Geometry: final body of the model. Coordinates: model frame, mm. Give positions to 0.01 mm unless a question says otherwise; leave off trailing zeros. Write each loop counter-clockwise with the first axis right and the second up, starting at its lowest first coordinate (ties: lowest second). Pieces come first, ordered by that corner, then holes. Notation, with made-up numbers: (-35, -25) -> (13, -25) arc R21 cw to (13, -17) -> close; hole circle Ø10 at (-4, -12.5). An arc over 180 degrees is marked (long way). Answer as a JSON object with one key per item and string values.
from build123d import *

# Parameters (mm, degrees)
SKETCH1_R           = 3.175
BOSS_EXTRUDE1_DEPTH = 3.175
SKETCH2_R           = 3.2004
SKETCH2_R_2         = 2.4384
CUT_EXTRUDE2_DEPTH  = 204.621243059
SKETCH3_R           = 4.73075
CUT_EXTRUDE3_DEPTH  = 1.5875
SKETCH5_R           = 0.9525
CUT_EXTRUDE4_DEPTH  = 204.621243059


with BuildPart() as part:
    # Sketch1 → Boss-Extrude1 (new body)
    with BuildSketch(Plane(origin=(0, 0, 0), x_dir=(0, 0, -1), z_dir=(1, 0, 0))):
        with BuildLine():
            Line((12.7, 12.7), (0, 12.7))
            ThreePointArc((0, 12.7), (-12.7, 0), (0, -12.7))
            Line((0, -12.7), (12.7, -12.7))
            Line((12.7, -12.7), (12.7, -9.525))
            Line((12.7, -9.525), (25.4, -9.525))
            Line((25.4, -9.525), (25.4, -12.7))
            Line((25.4, -12.7), (38.1, -12.7))
            Line((38.1, -12.7), (38.1, -9.525))
            Line((38.1, -9.525), (50.8, -9.525))
            Line((50.8, -9.525), (50.8, -12.7))
            Line((50.8, -12.7), (63.5, -12.7))
            Line((63.5, -12.7), (63.5, -9.525))
            Line((63.5, -9.525), (76.2, -9.525))
            Line((76.2, -9.525), (76.2, -12.7))
            Line((76.2, -12.7), (88.9, -12.7))
            Line((88.9, -12.7), (88.9, -9.525))
            Line((88.9, -9.525), (101.6, -9.525))
            Line((101.6, -9.525), (101.6, -12.7))
            Line((101.6, -12.7), (114.3, -12.7))
            Line((114.3, -12.7), (114.3, -9.525))
            Line((114.3, -9.525), (127, -9.525))
            Line((127, -9.525), (127, -12.7))
            Line((127, -12.7), (139.7, -12.7))
            Line((139.7, -12.7), (139.7, -9.525))
            Line((139.7, -9.525), (152.4, -9.525))
            Line((152.4, -9.525), (152.4, -12.7))
            Line((152.4, -12.7), (165.1, -12.7))
            Line((165.1, -12.7), (165.1, -9.525))
            Line((165.1, -9.525), (177.8, -9.525))
            Line((177.8, -9.525), (177.8, -12.7))
            Line((177.8, -12.7), (190.5, -12.7))
            Line((190.5, -12.7), (190.5, -9.525))
            Line((190.5, -9.525), (203.2, -9.525))
            Line((203.2, -9.525), (203.2, 9.525))
            Line((203.2, 9.525), (190.5, 9.525))
            Line((190.5, 9.525), (190.5, 12.7))
            Line((190.5, 12.7), (177.8, 12.7))
            Line((177.8, 12.7), (177.8, 9.525))
            Line((177.8, 9.525), (165.1, 9.525))
            Line((165.1, 9.525), (165.1, 12.7))
            Line((165.1, 12.7), (152.4, 12.7))
            Line((152.4, 12.7), (152.4, 9.525))
            Line((152.4, 9.525), (139.7, 9.525))
            Line((139.7, 9.525), (139.7, 12.7))
            Line((139.7, 12.7), (127, 12.7))
            Line((127, 12.7), (127, 9.525))
            Line((127, 9.525), (114.3, 9.525))
            Line((114.3, 9.525), (114.3, 12.7))
            Line((114.3, 12.7), (101.6, 12.7))
            Line((101.6, 12.7), (101.6, 9.525))
            Line((101.6, 9.525), (88.9, 9.525))
            Line((88.9, 9.525), (88.9, 12.7))
            Line((88.9, 12.7), (76.2, 12.7))
            Line((76.2, 12.7), (76.2, 9.525))
            Line((76.2, 9.525), (63.5, 9.525))
            Line((63.5, 9.525), (63.5, 12.7))
            Line((63.5, 12.7), (50.8, 12.7))
            Line((50.8, 12.7), (50.8, 9.525))
            Line((50.8, 9.525), (38.1, 9.525))
            Line((38.1, 9.525), (38.1, 12.7))
            Line((38.1, 12.7), (25.4, 12.7))
            Line((25.4, 12.7), (25.4, 9.525))
            Line((25.4, 9.525), (12.7, 9.525))
            Line((12.7, 9.525), (12.7, 12.7))
        make_face()
        Circle(SKETCH1_R, mode=Mode.SUBTRACT)
    extrude(amount=BOSS_EXTRUDE1_DEPTH)

    # Sketch2 → Cut-Extrude2 (cut, through all)
    with BuildSketch(Plane(origin=(3.175, 0, 0), x_dir=(0, 0, -1), z_dir=(1, 0, 0))):
        with Locations((15.875, 0)):
            Circle(SKETCH2_R)
        with Locations((187.325, 0)):
            Circle(SKETCH2_R_2)
    extrude(amount=-CUT_EXTRUDE2_DEPTH, mode=Mode.SUBTRACT)

    # Sketch3 → Cut-Extrude3 (cut)
    with BuildSketch(Plane(origin=(3.175, 0, 0), x_dir=(0, 0, -1), z_dir=(1, 0, 0))):
        with Locations((15.875, 0)):
            Circle(SKETCH3_R)
        Polygon((3.688171255, -6.3881), (7.376342509, 0), (3.688171255, 6.3881), (-3.688171255, 6.3881), (-7.376342509, 0), (-3.688171255, -6.3881), align=None)
    extrude(amount=-CUT_EXTRUDE3_DEPTH, mode=Mode.SUBTRACT)

    # Sketch5 → Cut-Extrude4 (cut, through all)
    with BuildSketch(Plane(origin=(3.175, 0, 0), x_dir=(0, 0, -1), z_dir=(1, 0, 0))):
        with Locations((-5.450627375, 0)):
            Circle(SKETCH5_R)
        with Locations((4.074372625, 0)):
            Circle(SKETCH5_R)
    extrude(amount=-CUT_EXTRUDE4_DEPTH, mode=Mode.SUBTRACT)


solid = part.part
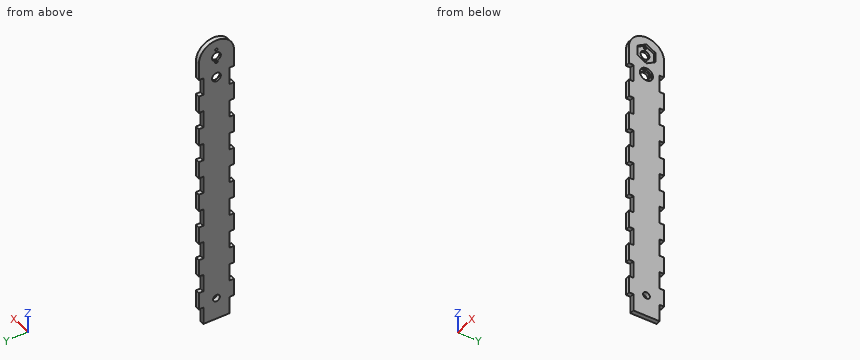
Q1. First-contact query: P1, Ø10, axis at y = 0, z = -131.5, coming from the -X side; P2, Ø1.6, axis at x = 2, z = -123.5, coming from the +Y side (3 decimals). Flat tips, straight axial feed; report the tip coordinate or a pass-through.
Values:
{"P1": "x = 0", "P2": "y = 9.525"}
Q2. Cut plane B-B (x = 2.55). State how many separate pieces and enclosed holes the cut face has, and give its area (3 significant figures).
Values:
{"separate pieces": "1", "enclosed holes": "3", "area": "4,540 mm²"}
Q3. Material intervals for L1, parallel to Y at x = 1.5, z = 0.5; L2, parallel to Y at x = 0.8, z = -24.5 (3 decimals); L3, parallel to Z at x = 2.2, y = -3.25, sorted ascending. Write a range as from..to.
Values:
{"L1": "-12.69..-3.14, 3.14..12.69", "L2": "-9.525..9.525", "L3": "-203.2..-19.31, -12.44..-5.5, 5.5..12.28"}
Q4. Cut plane A-A (z = -169). Return the cut outline in (x, y) (3 decimals).
Values:
{"outline": "(0, -9.525) -> (3.175, -9.525) -> (3.175, 9.525) -> (0, 9.525) -> close"}
